```python
from build123d import *

# Parameters (mm, degrees)
SKETCH1_W           = 10
SKETCH1_H           = 7
BOSS_EXTRUDE1_DEPTH = 12
SKETCH2_W           = 3
SKETCH2_H           = 7
CUT_EXTRUDE1_DEPTH  = 10
SKETCH3_R           = 2.125
CUT_EXTRUDE2_DEPTH  = 11


with BuildPart() as part:
    # Sketch1 → Boss-Extrude1 (new body)
    with BuildSketch(Plane(origin=(0, 0, 0), x_dir=(1, 0, 0), z_dir=(0, 1, 0))):
        with Locations((5, 3.5)):
            Rectangle(SKETCH1_W, SKETCH1_H)
    extrude(amount=BOSS_EXTRUDE1_DEPTH)

    # Sketch2 → Cut-Extrude1 (cut)
    with BuildSketch(Plane(origin=(0, 12, 0), x_dir=(1, 0, 0), z_dir=(0, 1, 0))):
        with Locations((3.5, 3.5)):
            Rectangle(SKETCH2_W, SKETCH2_H)
        with Locations((6.5, 3.5)):
            Rectangle(SKETCH2_W, SKETCH2_H)
    extrude(amount=-CUT_EXTRUDE1_DEPTH, mode=Mode.SUBTRACT)

    # Sketch3 → Cut-Extrude2 (cut, through all)
    with BuildSketch(Plane(origin=(10, 0, 0), x_dir=(0, 0, -1), z_dir=(1, 0, 0))):
        with Locations((3.5, 8)):
            Circle(SKETCH3_R)
    extrude(amount=-CUT_EXTRUDE2_DEPTH, mode=Mode.SUBTRACT)


solid = part.part
```
Model file for the job. Use its own axes, mm. A direction names the side the tool comes from. Coordinates: 2 decimals unless noted, no trailing zeros. Loops run counter-clockwise (first coordinate to the right, second up) from the corner with the lowest first, then second, coordinate; pieces in that order, holes last. Notation, with made-up numbers: (-26, 22) - (13, 22) arc R15 cw to (13, 30) - close; hole circle Ø6 at (64.25, 61). An arc over 180 degrees is marked (long way). Answer as a JSON object with one key per item and string values. Group by question number.
(1) Probe line 1 along X through (y, z) = (8.75, -1); line 2 along Y through (x, z) = (0.5, -3.5) (3 decimals); line 3 along Y through (x, z) = (7.25, -3.5). List the from-to ranges inside material, lowest first.
(2) Cut at D-D (x = 0.5). Give the cut face in (y, z) (3 decimals), then the cut area to 3 significant figures.
(3) Cut at C-C (y = 2.5). Give the cut face in (x, z).
(4) Cut at B-B (z = -3.5). Give the cut face in (x, y) (3 decimals).
(5) Tool access for faces 5 (the face through (1.6, 4.6, 0)), 6 (the face through (2, 6, -2)): list every direction of +Z, -Z, +X, -X, +Y, -Y with a clear straight run to the whole face (end or side of a thin tool).
(6) Two-plate mould, pull along Z, no slides. Class faces 1 (the face through (5, 2, -4)), 2 (the face through (9.01, 6.71, -1.81)), 3 (the face through (1.6, 4.6, -7)), 4 (the face through (1.01, 6.71, -1.81)): released by +Z, released by -Z, zero draft, split by the parting line, or undercut.
(7) Flat gauge pins, fed straight in: pin 1 (4 mm diameter, centred on y = 4.5, z = -6, fed in from -X); pin 2 (3 mm diameter, centred on x = 4, z = -5, fed in from +Y). Where does each tip first touch, or does it go through?
(8) Cut at A-A (y = 8). Give the cut face in (x, z) (3 decimals), then the cut area to 3 significant figures.
Geometry says:
{
 "1": {"line 1": "x = 0 to 2, 8 to 10", "line 2": "y = 0 to 5.875, 10.125 to 12", "line 3": "y = 0 to 2"},
 "2": {"outline": "(0, -7) - (12, -7) - (12, 0) - (0, 0) - close; hole circle Ø4.25 at (8, -3.5)", "area": "69.8 mm^2"},
 "3": {"outline": "(0, -7) - (2, -7) - (2, 0) - (0, 0) - close; (8, -7) - (10, -7) - (10, 0) - (8, 0) - close"},
 "4": {"outline": "(0, 0) - (10, 0) - (10, 5.875) - (8, 5.875) - (8, 2) - (2, 2) - (2, 5.875) - (0, 5.875) - close; (0, 10.125) - (2, 10.125) - (2, 12) - (0, 12) - close; (8, 10.125) - (10, 10.125) - (10, 12) - (8, 12) - close"},
 "5": {"face 5": "+Z, +X, -X, +Y, -Y", "face 6": "+Z, -Z, +Y"},
 "6": {"face 1": "zero draft", "face 2": "undercut", "face 3": "released by -Z", "face 4": "undercut"},
 "7": {"pin 1": "stops at x = 0", "pin 2": "stops at y = 2"},
 "8": {"outline": "(0, -7) - (2, -7) - (2, -5.625) - (0, -5.625) - close; (0, -1.375) - (2, -1.375) - (2, 0) - (0, 0) - close; (8, -7) - (10, -7) - (10, -5.625) - (8, -5.625) - close; (8, -1.375) - (10, -1.375) - (10, 0) - (8, 0) - close", "area": "11.0 mm^2"}
}
